```python
from build123d import *

# Parameters (mm, degrees)
BOSS_EXTRUDE1_DEPTH = 3
SKETCH2_R           = 2
BOSS_EXTRUDE2_DEPTH = 16
CHAMFER1_SIZE       = 0.25


with BuildPart() as part:
    # Sketch1 → Boss-Extrude1 (new body)
    with BuildSketch(Plane(origin=(0, 0, 0), x_dir=(1, 0, 0), z_dir=(0, 1, 0))):
        Polygon((4.618802154, 0), (2.309401077, 4), (-2.309401077, 4), (-4.618802154, 0), (-2.309401077, -4), (2.309401077, -4), align=None)
    extrude(amount=-BOSS_EXTRUDE1_DEPTH)

    # Sketch2 → Boss-Extrude2 (add)
    with BuildSketch(Plane(origin=(0, 0, 0), x_dir=(1, 0, 0), z_dir=(0, 1, 0))):
        with Locations(Location((0, 0, 0), (0, 0, 270))):
            Circle(SKETCH2_R)
    extrude(amount=BOSS_EXTRUDE2_DEPTH)

    # Chamfer1
    chamfer1_edges = [part.edges().sort_by_distance(p)[0] for p in [
        (0, 16, -2),
    ]]
    chamfer(chamfer1_edges, length=CHAMFER1_SIZE)


solid = part.part
```
Input: part model. Units: mm. Frame: model coordinates. A direction names the side the tool comes from. Round coordinates to 2 decimals unless told otherwise and drop trailing zeros. Order: outer loops, then holes, each group sorted by start corner. A loop starts at its lowest first (then second) coordinate and runs counter-clockwise, first axis right, second up. Notation, with made-up numbers: (71.5, 49) - (86.5, 49) arc R5 ccw to (86.5, 54) - close; hole circle Ø2 at (-37.5, 63). An arc over 180 degrees is marked (long way). One line per question, with ' | ' between items. Start each with the question number.
1) Contact query for flat-ended pins moving along their axis: P1, Ø5, axis at x = 2, y = 8, coming from the +Z side; P2, Ø1.5, axis at y = 0.5, z = 1.5, coming from the +X side; P3, Ø1.5, axis at y = 14, z = 3, coming from the +X side; P4, Ø3, axis at x = -2.5, z = 3, coming from the +Y side. Output: stop coordinate, or through.
2) Cut plane A-A, the plane x = 0. Return the cut outline in (y, z), then the cut area to 3 significant figures.
3) Set-up query: faces 1 (the cylindrical face through (-2, 8, 0)), 2 (the flat face through (3.448, -1.479, 2.028)). Return all of +Z, -Z, +X, -X, +Y, -Y with unobstructed straight access to the full face (end or side cutting, diameter ignored); none if empty.
4) Cut plane B-B, the plane y = -1.25. Return the cut outline in (x, z).
5) Cut plane D-D, the plane y = 9.75. Return the cut outline in (x, z).
6) Ray query, probe 1 along Y at (x, z) = (-3, 0); probe 2 along Z at (x, y) = (0.25, 1.75); probe 3 along X at (y, z) = (11, -1). Return the intervals inside material, ascending.
7) Cut plane C-C, the plane z = -2.5. Return the cut outline in (x, y), then the cut area to 3 significant figures.
Worked out:
1) P1: stops at z = 2 | P2: stops at x = 4.08 | P3: passes through | P4: stops at y = 0
2) outline: (-3, -4) - (0, -4) - (0, -2) - (15.75, -2) - (16, -1.75) - (16, 1.75) - (15.75, 2) - (0, 2) - (0, 4) - (-3, 4) - close | area: 87.9 mm^2
3) face 1: +Y | face 2: +Z, +X, +Y, -Y
4) outline: (-4.62, 0) - (-2.31, -4) - (2.31, -4) - (4.62, 0) - (2.31, 4) - (-2.31, 4) - close
5) outline: circle Ø4 at (0, 0)
6) probe 1: y = -3 to 0 | probe 2: z = -1.98 to 1.98 | probe 3: x = -1.73 to 1.73
7) outline: (-3.18, -3) - (3.18, -3) - (3.18, 0) - (-3.18, 0) - close | area: 19.1 mm^2
